Check sheet for the drawn part. Datum: minimum x, y, z corner. Units: mm. A direction names the side the tool comes from. Coordinates: 2 decimals unless noted, no trailing zeros. Write each loop counter-clockwise with the first axis right and the second up, starting at its lowest first coordinate (ties: lowest second). Pieces come first, ordered by that corner, then holes. Notation, with made-up numbers: (-14, -19.75) -> (26, -19.75) arc R9 cw to (26, -5.75) -> close; hole circle Ø4 at (25, 86.5). An arc over 180 degrees is marked (long way). Answer in a Markdown table with one row per item.
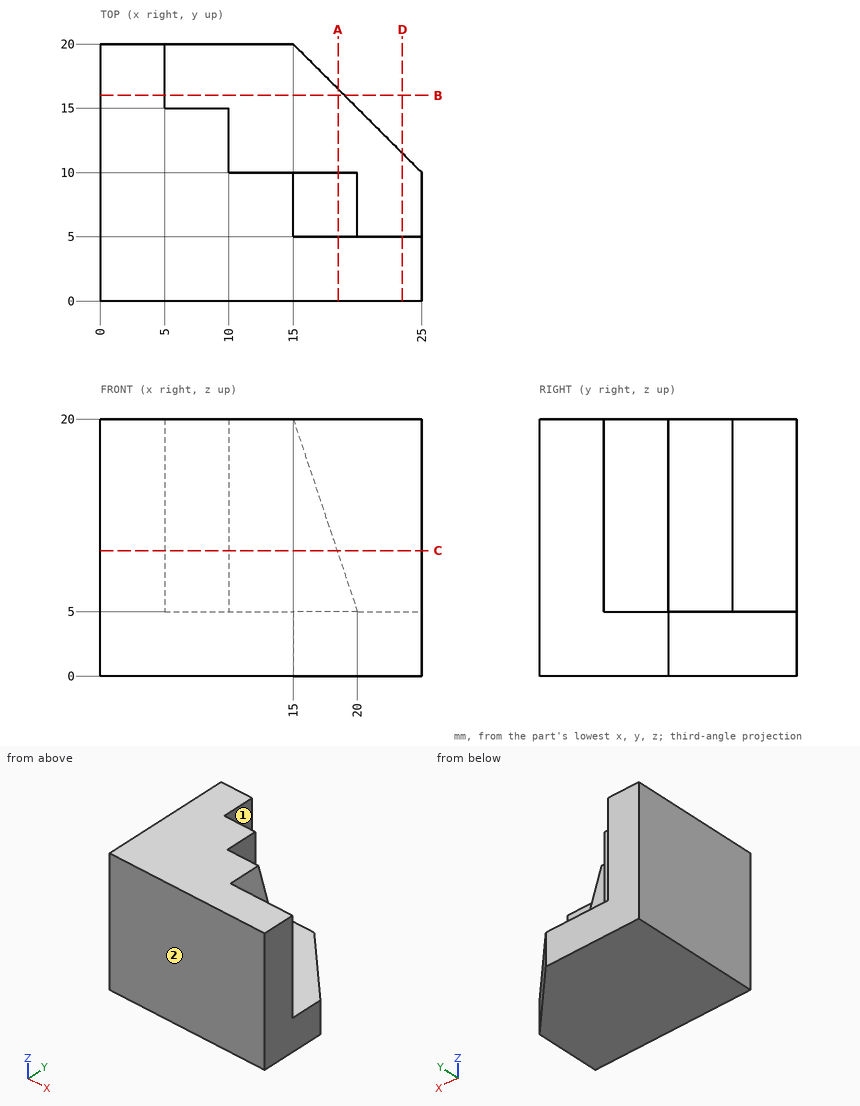
1. Sectioned sample at C-C, the plane z = 9.75. Record the cut outline in (x, y).
Findings below:
| item | result |
|---|---|
| outline | (0, 0) -> (25, 0) -> (25, 5) -> (18.42, 5) -> (18.42, 10) -> (10, 10) -> (10, 15) -> (5, 15) -> (5, 20) -> (0, 20) -> close |
2. Material ranges on probe 1 along Z at (x, y) = (13.25, 12.25); probe 2 along Y at (x, z) = (9.75, 6.5), recorded low to high. Write a range as from..to.
Findings below:
| item | result |
|---|---|
| probe 1 | z = 0..5 |
| probe 2 | y = 0..15 |
3. Access from +Z, -Z, +X, -X, +Y, -Y to the whole of each face (thin tool, end or side, straight path). Record for the marked faces 1 and 2.
Findings below:
| item | result |
|---|---|
| face 1 | +Z, +X, +Y |
| face 2 | +Z, -Z, +X, -X, -Y |
4. Sectioned sample at A-A, the plane x = 18.5. Record the cut outline in (y, z).
Findings below:
| item | result |
|---|---|
| outline | (0, 0) -> (16.5, 0) -> (16.5, 5) -> (10, 5) -> (10, 9.5) -> (5, 9.5) -> (5, 20) -> (0, 20) -> close |
5. Sectioned sample at B-B, the plane y = 16. Record the cut outline in (x, z), and give its area (3 significant figures).
Findings below:
| item | result |
|---|---|
| outline | (0, 0) -> (19, 0) -> (19, 5) -> (5, 5) -> (5, 20) -> (0, 20) -> close |
| area | 170 mm² |
6. Go/stop test with flat-tipped pins: pin 1 (5 mm diameter, centred on x = 17.5, z = 11.5, fed in from +Y); pin 2 (1.5 mm diameter, centred on x = 6.5, z = 11.5, fed in from +Y); pin 3 (1.5 mm diameter, centred on x = 19.5, y = 11, fed in from +Z). Record where each tip stops, or that it passes through.
Findings below:
| item | result |
|---|---|
| pin 1 | stops at y = 10 |
| pin 2 | stops at y = 15 |
| pin 3 | stops at z = 5 |
7. Sectioned sample at D-D, the plane x = 23.5. Record the cut outline in (y, z).
Findings below:
| item | result |
|---|---|
| outline | (0, 0) -> (11.5, 0) -> (11.5, 5) -> (5, 5) -> (5, 20) -> (0, 20) -> close |
